```python
from build123d import *

# Parameters (mm, degrees)
EXTRUDE_THIN1_DEPTH     = 166.6875
FILLET1_R               = 0.889
CUT_EXTRUDE1_DEPTH      = 1
CUT_EXTRUDE1_DEPTH_BACK = 167.6875


with BuildPart() as part:
    # Sketch1 → Extrude-Thin1 (new body)
    with BuildSketch(Plane.XY):
        with BuildLine():
            Line((0, 16.66875), (-3.125784133, 15.875))
            ThreePointArc((-3.125784133, 15.875), (-10.024656066, 11.362871681), (-12.7, 3.565675341))
            Line((-12.7, 3.565675341), (-12.7, 0))
            Line((-12.7, 0), (0, 0))
            Line((0, 0), (0, 0.889))
            Line((0, 0.889), (-11.811, 0.889))
            Line((-11.811, 0.889), (-11.811, 3.565675341))
            ThreePointArc((-11.811, 3.565675341), (-9.322930142, 10.817067937), (-2.906979244, 15.013347274))
            Line((-2.906979244, 15.013347274), (0.218804889, 15.807097274))
            Line((0.218804889, 15.807097274), (0, 16.66875))
        make_face()
    extrude(amount=-EXTRUDE_THIN1_DEPTH)

    # Fillet1
    fillet1_edges = [part.edges().sort_by_distance(p)[0] for p in [
        (-12.7, 0, -83.34375),
    ]]
    fillet(fillet1_edges, radius=FILLET1_R)

    # Sketch2 → Cut-Extrude1 (cut, two sides)
    with BuildSketch(Plane.XY) as cut_extrude1_sk:
        Polygon((0, -55.634586178), (0, 0.889), (0, 19.48899735), (0, 76.012583528), (113.047172356, 76.012583528), (113.047172356, -55.634586178), align=None)
    extrude(amount=CUT_EXTRUDE1_DEPTH, mode=Mode.SUBTRACT)
    extrude(cut_extrude1_sk.sketch, amount=-CUT_EXTRUDE1_DEPTH_BACK, mode=Mode.SUBTRACT)


solid = part.part
```
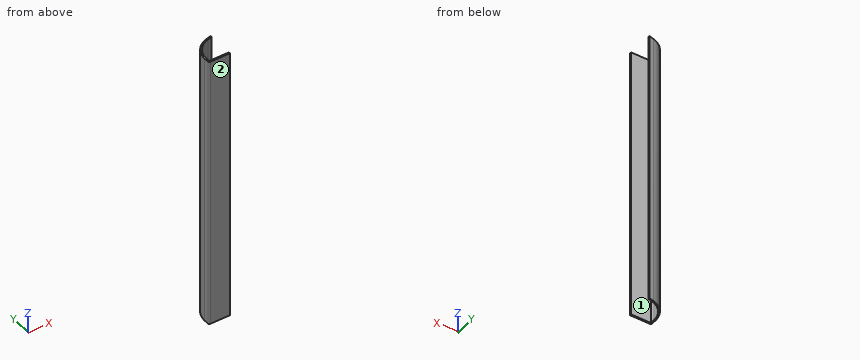
Work out the finished part from the listing and answer in its coordinate system (mm). Face numbers are marked on the shaded views. Give positions to 0.01 mm unless a question says otherwise; leave off trailing zeros. Loops run counter-clockwise (first coordinate to the right, second up) from the corner with the lowest first, then second, coordinate; pieces in that order, holes last. Notation, with made-up numbers: (3, 60) - (49, 60) arc R16 cw to (49, 82) - close; hole circle Ø10 at (80, -3.5). An arc over 180 degrees is marked (long way). Use CSV: the item, a comma, the result in double quotes. Start each with the question number.
(1) Find the intervals of material crossed by L1, parallel to Y at x = -3, z = -15; L2, parallel to Y at x = -8, z = -72.5; L3, parallel to X at y = 1.75, z = -104.5, in increasing order.
(2) Each of these flat-tipped pins is pushed along its axis until it touches: pin 1 (1 mm diameter, centred on y = 9, z = -101, fed in from -X); pin 2 (3 mm diameter, centred on y = 2.5, z = -83.5, fed in from +X); pin 3 (3.5 mm diameter, centred on x = -4.5, z = -48.5, fed in from +Y). Where does it stop, or does it pass through?
(3) Find section B-B, the plane z = -59.5. Determine the outline of the cut face in (x, y) (3 decimals), plus the area to 3 significant figures.
(4) Find section A-A, the plane x = -8.75. Determine the outline of the cut face in (y, z), plus the area to 3 significant figures.
(5) Find section C-C, the plane y = 9. Determine the outline of the cut face in (x, z), plus the area to 3 significant figures.
(6) Determine the mould class of the marked faces 1 and 2 for opening direction Y: released by +Y, released by -Y, zero draft, split by the parting line, or undercut.
Results found:
1,L1,"0 to 0.89, 14.99 to 15.91"
1,L2,"0 to 0.89, 12.25 to 13.43"
1,L3,"-12.7 to -11.81"
2,pin 1,"x = -11.7"
2,pin 2,"x = -11.8"
2,pin 3,"y = 15.97"
3,outline,"(-12.7, 0.889) arc R0.889 ccw to (-11.811, 0) - (0, 0) - (0, 0.889) - (-11.811, 0.889) - (-11.811, 3.566) arc R11.811 cw to (-2.907, 15.013) - (0, 15.752) - (0, 16.669) - (-3.126, 15.875) arc R12.7 ccw to (-12.7, 3.566) - close"
3,area,"30.7 mm^2"
4,outline,"(0, -166.69) - (0.89, -166.69) - (0.89, 0) - (0, 0) - close; (11.5, -166.69) - (12.77, -166.69) - (12.77, 0) - (11.5, 0) - close"
4,area,"360 mm^2"
5,outline,"(-11.48, -166.69) - (-10.49, -166.69) - (-10.49, 0) - (-11.48, 0) - close"
5,area,"165 mm^2"
6,face 1,"undercut"
6,face 2,"released by -Y"
